Autodesk Inventor part; units mm, degrees
ref_plane "YZ Plane" through (0, 0, 0) normal (1, 0, 0) x (0, 1, 0)
ref_plane "XZ Plane" through (0, 0, 0) normal (0, 1, 0) x (-1, 0, 0)
ref_plane "XY Plane" through (0, 0, 0) normal (0, 0, 1) x (1, 0, 0)
sketch "Sketch1" plane through (0, 0, 0) normal (0, 1, 0) x (-1, 0, 0)
  circle A0 centre (-7.366, 0) radius 1.143
  circle A1 centre (7.366, 0) radius 1.143
  line L0 (10.16, 0) -> (10.16, 0)
  line L1 (10.16, 0) -> (10.16, 0)
  line L2 (-10.16, 0) -> (-10.16, 0)
  line L3 (-10.16, 0) -> (-10.16, 0)
  arc A2 (-10.16, 0) -> (-7.62, -2.54) centre (-7.62, 0) ccw
  arc A3 (-7.8454, 2.53) -> (-10.16, 0) centre (-7.62, 0) ccw
  arc A4 (10.16, 0) -> (7.8454, 2.53) centre (7.62, 0) ccw
  arc A5 (7.8454, -2.53) -> (10.16, 0) centre (7.62, 0) ccw
  arc A6 (7.8454, 2.53) -> (-7.8454, 2.53) centre (0, 0) ccw
  arc A7 (-7.8454, -2.53) -> (7.8454, -2.53) centre (0, 0) ccw
  dimension "d2" = 2.286
  dimension "d15" = 2.54
  dimension "d16" = 2.54
  dimension "d17" = 2.54
extrude "Extrusion1" add sketch "Sketch1" along normal blind 0.762
sketch "Sketch2" plane through (0, 0.762, 0) normal (0, 1, 0) x (1, 0, 0)
  point P0 (0, 0)
sketch "Sketch3" plane through (0, 0.762, 0) normal (0, 1, 0) x (1, 0, 0)
  line L0 (-7.2575, -1.2599) -> (-7.2559, -1.2599)
  line L1 (-7.2559, -1.2599) -> (-7.2559, -1.269)
  line L2 (-7.1482, -1.778) -> (-6.096, -1.778)
  line L3 (-7.2559, 1.269) -> (-7.2559, 1.27)
  line L4 (-7.1482, 1.778) -> (-6.096, 1.778)
  arc A0 (7.1482, 1.778) -> (-7.1482, 1.778) centre (0, 0) ccw
  arc A1 (-7.2557, 1.27) -> (-7.2559, 1.269) centre (0, 0) ccw
  arc A2 (-7.2575, -1.2599) -> (-7.2559, -1.269) centre (0, 0) ccw
  arc A3 (-7.1482, -1.778) -> (7.1482, -1.778) centre (0, 0) ccw
  line L5 (-7.2575, -1.2599) -> (-7.2559, -1.2599)
  line L6 (6.096, -1.778) -> (7.1482, -1.778)
  line L7 (6.096, 1.778) -> (7.1482, 1.778)
  arc A4 (6.096, 1.778) -> (-6.096, 1.778) centre (0, 0) ccw
  arc A5 (-6.096, -1.778) -> (6.096, -1.778) centre (0, 0) ccw
extrude "Extrusion2" add sketch "Sketch3" along normal blind 7.62 contours A0 L7 A4 L4 | L2 A5 L6 A1
fillet "Fillet1" radius 1.27 4 edges at (6.6221, 8.382, 1.778) (-6.6221, 8.382, 1.778) (-6.6221, 8.382, -1.778) (6.6221, 8.382, -1.778)
fillet "Fillet2" radius 0.508 10 edges at (5.9835, 7.9854, -2.126) (6.096, 3.937, -1.778) (-5.9838, 7.9847, -2.1254) (-6.096, 3.937, -1.778) (0, 8.382, -6.35) (-5.9835, 7.9854, 2.126) (-6.096, 3.937, 1.778) (5.9835, 7.9854, 2.126) (6.096, 3.937, 1.778) (0, 8.382, 6.35)
properties part number "polulu_caster"
Geometry: final body of the model. Coordinates: model frame, mm. A direction names the side the tool comes from. Coordinates: 2 decimals unless noted, no trailing zeros. Write each loop counter-clockwise with the first axis right and the second up, starting at its lowest first coordinate (ties: lowest second). Pieces come first, ordered by that corner, then holes. Notation, with made-up numbers: M 25,15 L 55,15 A14 ccw 55,24 Z; hole C -39,44 d6. An arc over 180 degrees is marked long. Answer as CSV lines item,"result". Start each with the question number.
Q1. Mould query, pull axis X, two halves, no side actions, for faces 1 (the cylindrical face through (0.137, 4.519, 7.365)), 2 (the flat face through (0, 0, 0)), 3 (the flat face through (0, 0.762, 0)), 4 (the cylindrical face through (0.11, 4.27, 6.35)). Classes: released by +X, released by -X, zero draft, split by the parting line, or undercut.
Q2. Cut plane C-C on z = 0.25. Return the cut outline in (x, y).
Q3. Cut plane B-B on x = 7.5. Return the cut outline in (y, z).
Q4. Cut plane A-A on y = 2. Return the cut outline in (x, z).
Q5. Pin query (flat end, axial travel): P1, Ø3, axis at x = 2, z = 0, coming from the +Y side; P2, Ø1.5, axis at x = 4, y = 3.5, coming from the -Z side; P3, Ø0.8, axis at x = -7, y = 3.5, coming from the -Z side; P4, Ø2, axis at x = 7.366, z = 0, coming from the -Y side. Return the tip coordinate at first contact, or that it passes through.
Q6. Cut plane D-D on x = 0. Return the cut outline in (y, z), then the cut area to 3 significant figures.
Q7. Reachability of faces 5 (the cylindrical face through (-0.137, 4.519, -7.365)), 6 (the flat face through (-1, 8.382, 7)), 7 (the cylindrical face through (6.65, 8, 2.14)), 8 (the cylindrical face through (-0.11, 4.27, -6.35)) from +Z, -Z, +X, -X, +Y, -Y: full face, straight path, thin tool, end or side. Return the list, or none.
Q8. Line query: line 1 (Z direction, x = 6.25, y = 7.75); line 2 (Z direction, x = 0.5, y = 7.5); line 3 (X direction, y = 7.5, z = 3.75). Output: solid intervals per line, ascending. Write a range as from..to.
Findings below:
1,face 1,"split by the parting line"
1,face 2,"zero draft"
1,face 3,"undercut"
1,face 4,"undercut"
2,outline,"M -10.15,0 L -8.48,0 L -8.48,0.76 L -10.15,0.76 Z; M -6.25,0 L 6.25,0 L 6.25,0.76 L -6.25,0.76 Z; M 8.48,0 L 10.15,0 L 10.15,0.76 L 8.48,0.76 Z"
3,outline,"M 0,-3.42 L 0.76,-3.42 L 0.76,-1.14 L 0,-1.14 Z; M 0,1.14 L 0.76,1.14 L 0.76,3.42 L 0,3.42 Z"
4,outline,"M -7.15,-1.78 A7.37 ccw 7.15,-1.78 L 6.47,-1.78 A0.51 ccw 5.99,-2.12 A6.35 cw -5.99,-2.12 A0.51 ccw -6.47,-1.78 Z; M -7.15,1.78 L -6.47,1.78 A0.51 ccw -5.99,2.12 A6.35 cw 5.99,2.12 A0.51 ccw 6.47,1.78 L 7.15,1.78 A7.37 ccw Z"
5,P1,"stops at y = 0.76"
5,P2,"stops at z = -6.61"
5,P3,"stops at z = -3.27"
5,P4,"passes through"
6,outline,"M 0,-8.24 L 0.76,-8.24 L 0.76,-7.37 L 8.38,-7.37 L 8.38,-6.86 A0.51 ccw 7.87,-6.35 L 0.76,-6.35 L 0.76,6.35 L 7.87,6.35 A0.51 ccw 8.38,6.86 L 8.38,7.37 L 0.76,7.37 L 0.76,8.24 L 0,8.24 Z"
6,area,"27.9 mm2"
7,face 5,"-Z, +Y"
7,face 6,"+Z, -Z, +X, -X, +Y"
7,face 7,"+X, -X, +Y"
7,face 8,"+Y"
8,line 1,"z = -3.9..-1.98, 1.98..3.9"
8,line 2,"z = -7.35..-6.33, 6.33..7.35"
8,line 3,"x = -6.34..-5.12, 5.12..6.34"
